```python
from build123d import *

# Parameters (mm, degrees)
MODEL_R             = 1.5
MODEL_R_2           = 1
MODEL_R_3           = 3
BOSS_EXTRUDE1_DEPTH = 3


with BuildPart() as part:
    # Model → Boss-Extrude1 (new body)
    with BuildSketch(Plane.XY):
        Polygon((26.589929576, 98.91813413), (26.589929576, 45.61813413), (80.889929576, 45.61813413), (80.889929576, 12.26813413), (136.589929576, 12.26813413), (136.589929576, 45.61813413), (136.589929576, 98.91813413), align=None)
        with Locations((40.589929576, 96.41813413)):
            Circle(MODEL_R, mode=Mode.SUBTRACT)
        with Locations((92.689929576, 63.41813413)):
            Circle(MODEL_R, mode=Mode.SUBTRACT)
        with Locations((41.889929576, 48.21813413)):
            Circle(MODEL_R, mode=Mode.SUBTRACT)
        with Locations((92.689929576, 91.31813413)):
            Circle(MODEL_R, mode=Mode.SUBTRACT)
        with Locations((110.589929576, 39.76813413)):
            Circle(MODEL_R_2, mode=Mode.SUBTRACT)
        with Locations((46.589929576, 72.26813413)):
            Circle(MODEL_R_2, mode=Mode.SUBTRACT)
        with Locations((83.589929576, 72.26813413)):
            Circle(MODEL_R_2, mode=Mode.SUBTRACT)
        with Locations((132.589929576, 25.76813413)):
            Circle(MODEL_R_2, mode=Mode.SUBTRACT)
        with Locations((91.589929576, 23.91813413)):
            Circle(MODEL_R_3, mode=Mode.SUBTRACT)
        with Locations((132.589929576, 53.76813413)):
            Circle(MODEL_R_2, mode=Mode.SUBTRACT)
    extrude(amount=BOSS_EXTRUDE1_DEPTH)


solid = part.part
```
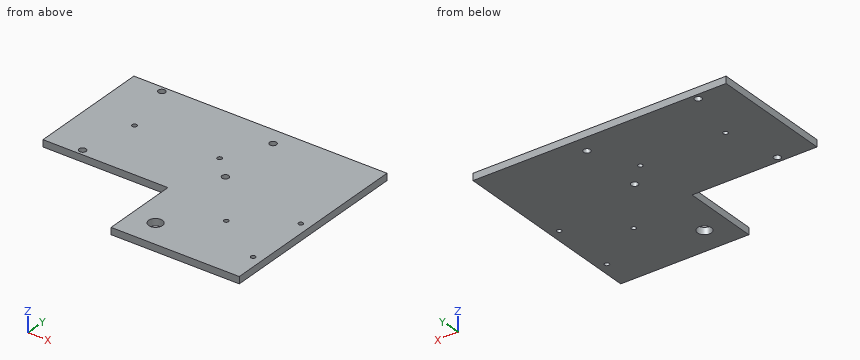
Model file for the job. Use its own axes, mm. Coordinates: 2 decimals unless noted, no trailing zeros. Order: outer loops, then holes, each group sorted by start corner. A loop starts at its lowest first (then second) coordinate and runs counter-clockwise, first axis right, second up. Notation, with made-up numbers: (29.5, -0.75) - (55.5, -0.75) arc R28 cw to (55.5, 17.25) - close; hole circle Ø11 at (59, 15). An arc over 180 degrees is marked (long way). Return JSON: item names as keys, results as strings. Group by question number.
1) Saw through at A-A, the plane x = 93. Write the cut outline in (y, z).
2) Probe line 1 (Y direction, x = 77, z = 1.15); line 2 (X direction, y = 29, z = 0.3); line 3 (X direction, y = 47, z = 2.7). List the from-to ranges inside material, lowest first. Write a range as from..to.
3) Saw through at C-C, the plane x = 66. Write the cut outline in (y, z), plus the area to 3 significant figures.
4) Flat gauge pin, fed straight in: P1, Ø0.9, axis at y = 21, z = 1, coming from the -X side. Where does the tip first touch, or does it go through?
5) Saw through at B-B, the plane z = 1.75. Count the separate pieces of the cut face and the enclosed holes in it, plus the area to 3 significant figures.
Values found:
{
 "1": {"outline": "(12.27, 0) - (21.27, 0) - (21.27, 3) - (12.27, 3) - close; (26.57, 0) - (61.95, 0) - (61.95, 3) - (26.57, 3) - close; (64.89, 0) - (89.85, 0) - (89.85, 3) - (64.89, 3) - close; (92.79, 0) - (98.92, 0) - (98.92, 3) - (92.79, 3) - close"},
 "2": {"line 1": "y = 45.62..98.92", "line 2": "x = 80.89..136.59", "line 3": "x = 26.59..41.01, 42.77..136.59"},
 "3": {"outline": "(45.62, 0) - (98.92, 0) - (98.92, 3) - (45.62, 3) - close", "area": "160 mm²"},
 "4": {"P1": "stops at x = 80.89"},
 "5": {"separate pieces": "1", "enclosed holes": "10", "area": "7,650 mm²"}
}
